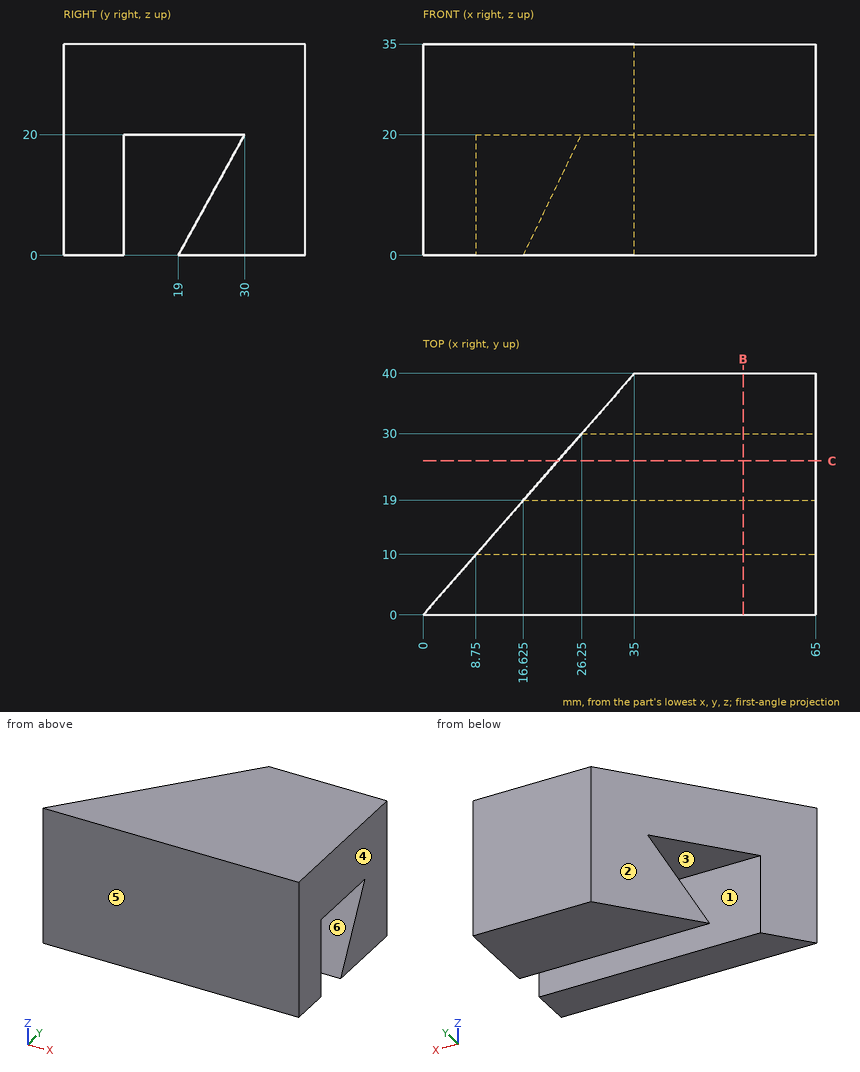
Here's the drawing with two shaded views (mm, measured from the low corner). I have some questions. A direction names the side the tool comes from. Give positions to 0.01 mm unless a question says otherwise; leave off trailing zeros. Loops run counter-clockwise (first coordinate to the right, second up) from the corner with the lowest first, then second, coordinate; pieces in that order, holes last. Notation, with made-up numbers: M -26.75,-10.5 L 26.25,-10.5 A30 ccw 26.25,22.5 Z; hole C 12.5,5.25 d2. An arc over 180 degrees is marked long. Use one line per item in the form item = value. Start each with the question number.
Q1. If we section it at C-C (y = 25.5): Write out the boundary of the cut face in (x, z).
Q2. Thinking about a two-plate mould opening in Y: for the marked faces 4, 5 and 6, which applies, +Y half, -Y half, draft (parallel to the pull), parting line (faces both ways), or undercut?
Q3. Will these pins go through, and if not, where does the flat tip stop? pin 1 Ø1 at (y, z) = (9.5, 7) entering from -X (3 decimals); pin 2 Ø8 at (x, z) = (16.5, 29) entering from +Y.
Q4. Which directions (+Z, -Z, +X, -X, +Y, -Y) give clear straight access to the entire face, cutting with the end or side of a thin tool? Please do the marked faces 1, 2 and 3.
Q5. I need wall thicknesses on line 1 along Y through (x, z) = (14, 4); line 2 along Z through (x, y) = (48, 19.5); line 3 along Z through (x, y) = (62, 20.5). Which ranges of each line are inside material? Lowest first, please.
Q6. If we section it at B-B (x = 53): Write out the boundary of the cut face in (y, z), then the cut area to 3 significant figures.
Taken from the geometry:
q1.outline = M 22.31,0 L 65,0 L 65,11.82 L 22.31,11.82 Z; M 22.31,20 L 65,20 L 65,35 L 22.31,35 Z
q2.face_4 = draft
q2.face_5 = -Y half
q2.face_6 = undercut
q3.pin_1 = 7.875
q3.pin_2 = 23.43
q4.face_1 = -Z, +X, -X
q4.face_2 = +Z, -Z, -X, +Y
q4.face_3 = +X, -X
q5.line_1 = 0 to 10
q5.line_2 = 0 to 0.91, 20 to 35
q5.line_3 = 0 to 2.73, 20 to 35
q6.outline = M 0,0 L 10,0 L 10,20 L 30,20 L 19,0 L 40,0 L 40,35 L 0,35 Z
q6.area = 1,110 mm^2
